```python
from build123d import *

# Parameters (mm, degrees)
F1_DEPTH  = 180
F4_W      = 2.5
F4_H      = 4
F5_DEPTH  = 164
F6_W      = 2.5
F6_H      = 2.5
F7_DEPTH  = 7.5
F8_W      = 10
F8_H      = 2.5
F9_DEPTH  = 25
F10_W     = 1.5
F10_H     = 1
F11_DEPTH = 170


with BuildPart() as f1:
    # F0 (on Front) → F1 (new body)
    with BuildSketch(Plane.XZ):
        Polygon((-149.2392462472, 9.4979269803), (-64.5789922093, 9.4979269803), (20.0812618285, 9.4979269803), (20.0812618285, 11.9979269803), (17.5812618285, 11.9979269803), (17.5812618285, 14.4979269803), (20.0812618285, 14.4979269803), (20.0812618285, 16.9979269803), (17.5812618285, 16.9979269803), (8.9210077907, 11.9979269803), (-64.5789922093, 11.9979269803), (-138.0789922093, 11.9979269803), (-146.7392462472, 16.9979269803), (-149.2392462472, 16.9979269803), (-149.2392462472, 14.4979269803), (-146.7392462472, 14.4979269803), (-146.7392462472, 11.9979269803), (-149.2392462472, 11.9979269803), align=None)
    extrude(amount=-F1_DEPTH)

    # F4 (on offset) → F5 (join)
    with BuildSketch(Plane(origin=(-146.7392462472, 0, 0), x_dir=(0, -1, 0), z_dir=(-1, 0, 0))):
        with Locations((-178.75, 11.4979269803)):
            Rectangle(F4_W, F4_H)
        with Locations((-134.375, 11.4979269803)):
            Rectangle(F4_W, F4_H)
        with Locations((-90, 11.4979269803)):
            Rectangle(F4_W, F4_H)
        with Locations((-45.625, 11.4979269803)):
            Rectangle(F4_W, F4_H)
        with Locations((-1.25, 11.4979269803)):
            Rectangle(F4_W, F4_H)
    extrude(amount=-F5_DEPTH)

    # F6 (on face) → F7 (join)
    with BuildSketch(Plane(origin=(0, 0, 9.4979269803), x_dir=(1, 0, 0), z_dir=(0, 0, -1))):
        with Locations((-147.9892462472, -1.25)):
            Rectangle(F6_W, F6_H)
        with Locations((18.8312618285, -1.25)):
            Rectangle(F6_W, F6_H)
        with Locations((18.8312618285, -178.75)):
            Rectangle(F6_W, F6_H)
        with Locations((-147.9892462472, -178.75)):
            Rectangle(F6_W, F6_H)
    extrude(amount=-F7_DEPTH)

    # F8 (on face) → F9 (cut)
    with BuildSketch(Plane.XY.offset(11.9979269803)):
        with Locations((-141.7392462472, 3.75)):
            Rectangle(F8_W, F8_H)
        with Locations((-141.7392462472, 176.25)):
            Rectangle(F8_W, F8_H)
        with Locations((12.5812618285, 176.25)):
            Rectangle(F8_W, F8_H)
        with Locations((12.5812618285, 3.75)):
            Rectangle(F8_W, F8_H)
    extrude(amount=F9_DEPTH, mode=Mode.SUBTRACT)

    # F10 (on face) → F11 (join)
    with BuildSketch(Plane(origin=(0, 175, 0), x_dir=(-1, 0, 0), z_dir=(0, 1, 0))):
        with Locations((135.8289922093, 12.4979269803)):
            Rectangle(F10_W, F10_H)
        with Locations((100.2039922093, 12.4979269803)):
            Rectangle(F10_W, F10_H)
        with Locations((64.5789922093, 12.4979269803)):
            Rectangle(F10_W, F10_H)
        with Locations((28.9539922093, 12.4979269803)):
            Rectangle(F10_W, F10_H)
        with Locations((-6.6710077907, 12.4979269803)):
            Rectangle(F10_W, F10_H)
    extrude(amount=-F11_DEPTH)


solid = f1.part
```
Source: CAD feature listing. Evaluate the final solid. Frame: model axes, mm. A direction names the side the tool comes from. Give positions to 0.01 mm unless a question says otherwise; leave off trailing zeros. Write each loop counter-clockwise with the first axis right and the second up, starting at its lowest first coordinate (ties: lowest second). Pieces come first, ordered by that corner, then holes. Notation, with made-up numbers: (87.25, 58.25) - (115.25, 58.25) arc R35 ccw to (115.25, 90.25) - close; hole circle Ø7 at (27, 30.25). An arc over 180 degrees is marked (long way). One line per item, written item: value. Start each with the question number.
Q1. Material intervals for probe 1 along Y at (x, z) = (-68, 12.25) (3 decimals); probe 2 along Z at (x, y) = (-2, 161.5); probe 3 along X at (y, z) = (44, 16), sorted ascending. Write a range as from..to.
Q2. First-contact query: pin 1 Ø1.5 at (x, y) = (-102, 138.5) entering from +Z; pin 2 Ø0.5 at (y, z) = (118, 12.5) entering from -X; pin 3 Ø1.5 at (y, z) = (106, 13) entering from +X; pin 4 Ø2.5 at (x, z) = (-57, 15.5) entering from +Y. Flat tips, straight axial feed; report the tip coordinate or a pass-through.
Q3. Set-up query: faces 4 (the face through (-66, 0, 12)), 5 (the face through (-143, 5, 14)). Return all of +Z, -Z, +X, -X, +Y, -Y with unobstructed straight access to the full face (end or side cutting, diameter ignored); none if empty.
Q4. Section query A-A, the plane x = -49. Return the cut outline in (y, z) (3 decimals), then the cut area to 3 significant figures.
Q5. Draft query along X for faces 1 (the face through (-66, 91, 9.498)), 2 (the face through (-82, 112, 11.998)), 3 (the face through (-149.239, 88.7, 11.6)). Return one class per face: +X half, -X half, draft (parallel to the pull), parting line (faces both ways), or undercut.
Answer:
1. probe 1: y = 0..2.5, 44.375..46.875, 88.75..91.25, 133.125..135.625, 177.5..180
1. probe 2: z = 9.5..12
1. probe 3: x = -149.24..-145.01, 15.85..20.08
2. pin 1: stops at z = 12
2. pin 2: stops at x = -146.74
2. pin 3: stops at x = 17.58
2. pin 4: passes through
3. face 4: +Z, -Z, +X, -X, -Y
3. face 5: +Z
4. outline: (0, 9.498) - (180, 9.498) - (180, 13.498) - (177.5, 13.498) - (177.5, 11.998) - (135.625, 11.998) - (135.625, 13.498) - (133.125, 13.498) - (133.125, 11.998) - (91.25, 11.998) - (91.25, 13.498) - (88.75, 13.498) - (88.75, 11.998) - (46.875, 11.998) - (46.875, 13.498) - (44.375, 13.498) - (44.375, 11.998) - (2.5, 11.998) - (2.5, 13.498) - (0, 13.498) - close
4. area: 469 mm2
5. face 1: draft
5. face 2: undercut
5. face 3: -X half
